Model file for the job. Use its own axes, mm. Face numbers are marked on the shaded views. A direction names the side the tool comes from. Coordinates: 2 decimals unless noted, no trailing zeros. Write each loop counter-clockwise with the first axis right and the second up, starting at its lowest first coordinate (ties: lowest second). Pieces come first, ordered by that corner, then holes.
Q1. Band-saw the part on A-A, the plane z = 1.75. Write the cut outline in (x, y).
Q2. Pull direction X, two halves, no side cores. Call the marked faces 1, 2, 3 and 4: released by +X, released by -X, zero draft, split by the parting line, or undercut.
Q3. Drill centre lines: probe 1 along X at (y, z) = (-16, 3.5); probe 2 along X at (y, z) = (10.5, 2.25); probe 3 along X at (y, z) = (7.5, 5.5). Where is each one in solid material? Low to high.
Q4. Pin check, flat tips, straight feed: P1, Ø1, axis at y = 1, z = 2, coming from the -X side; P2, Ø1.5, axis at x = -30, z = 2.5, coming from the -Y side; P3, Ø4, axis at x = 32, z = 3, coming from the -Y side; P4, Ø21, axis at x = -29.05, y = 0, coming from the +Z side. Stop position of each tip, or through.
Q5. Which spindle directions (+Z, -Z, +X, -X, +Y, -Y) get a long thin tool onto all of the face, cutting with end or side? Do the marked faces 5 and 6. Say none if no direction does.
Q6. Band-saw the part on C-C, the plane y = 0. Write the cut outline in (x, z), plus the area to 3 significant figures.
Q7. Band-saw the part on D-D, the plane x = -17. Write the cut outline in (y, z), plus the area to 3 significant figures.
Q8. Band-saw the part on B-B, the plane x = 35. Write the cut outline in (y, z).
from build123d import *

# Parameters (mm, degrees)
F0_R     = 13.2
F1_DEPTH = 7


with BuildPart() as f1:
    # F0 (on Top) → F1 (new body)
    with BuildSketch(Plane.XY):
        with BuildLine():
            ThreePointArc((5.644667, 22.165649), (4.665852, 19.88717), (3.409515, 17.749143))
            ThreePointArc((3.409515, 17.749143), (0.156216, 19.184844), (-3.20524, 18.024758))
            ThreePointArc((-3.20524, 18.024758), (-4.974394, 19.897283), (-6.195367, 22.165649))
            ThreePointArc((-6.195367, 22.165649), (-7.382922, 19.823517), (-8.993153, 17.749143))
            ThreePointArc((-8.993153, 17.749143), (-22.389875, 12.804904), (-33.179633, 22.158981))
            ThreePointArc((-33.179633, 22.158981), (-49.675616, 1.648765), (-33.179633, -18.861452))
            ThreePointArc((-33.179633, -18.861452), (-15.982306, -11.966628), (0, -21.339599))
            ThreePointArc((0, -21.339599), (18.241916, -11.616609), (36.483832, -21.339599))
            ThreePointArc((36.483832, -21.339599), (50.653593, 0.409691), (36.483832, 22.158981))
            ThreePointArc((36.483832, 22.158981), (23.994879, 12.812003), (9.197427, 17.749143))
            ThreePointArc((9.197427, 17.749143), (7.450629, 19.981192), (5.644667, 22.165649))
        make_face()
        with Locations((-29.049389, 0)):
            Circle(F0_R, mode=Mode.SUBTRACT)
        Circle(F0_R, mode=Mode.SUBTRACT)
        with Locations((29.32474, 0)):
            Circle(F0_R, mode=Mode.SUBTRACT)
    extrude(amount=F1_DEPTH)


solid = f1.part
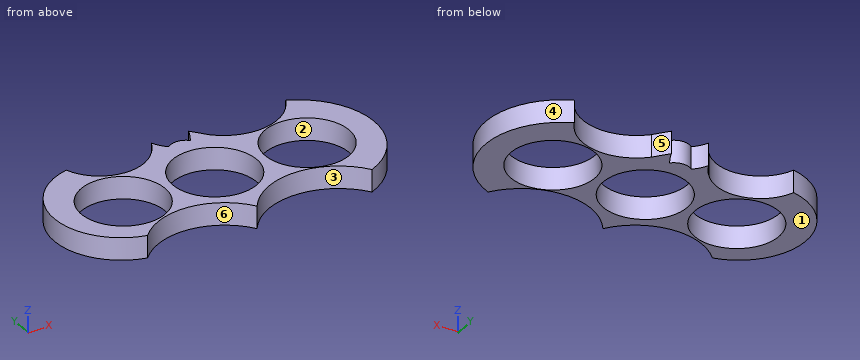
Answer sheet:
1. outline: (-33.18, -18.86) arc R21.04 cw to (0, -21.34) arc R21.97 cw to (36.48, -21.34) arc R23.78 ccw to (36.48, 22.16) arc R16.82 cw to (9.2, 17.75) arc R105.8 ccw to (5.64, 22.17) arc R19.77 cw to (3.41, 17.75) arc R4.87 ccw to (-3.21, 18.02) arc R9.81 cw to (-6.2, 22.17) arc R13.78 cw to (-8.99, 17.75) arc R14.03 cw to (-33.18, 22.16) arc R21 ccw to start; hole circle Ø26.4 at (-29.05, 0); hole circle Ø26.4 at (0, 0); hole circle Ø26.4 at (29.32, 0)
2. face 1: zero draft
2. face 2: undercut
2. face 3: undercut
2. face 4: released by +X
3. probe 1: x = -40.06 to -30.02, -5.08 to 5.07, 31.41 to 44.08
3. probe 2: x = -47.72 to -37.05, -21.05 to -8, 8 to 21.33, 37.32 to 48.41
3. probe 3: x = -48.84 to -39.91, -18.19 to -10.86, 10.86 to 18.46, 40.19 to 49.57
4. P1: stops at x = -49.68
4. P2: stops at y = -16.56
4. P3: stops at y = -18.28
4. P4: passes through
5. face 5: +Z, -Z, +Y
5. face 6: +Z, -Z, -Y
6. outline: (-49.61, 0) - (-42.25, 0) - (-42.25, 7) - (-49.61, 7) - close; (-15.85, 0) - (-13.2, 0) - (-13.2, 7) - (-15.85, 7) - close; (13.2, 0) - (16.12, 0) - (16.12, 7) - (13.2, 7) - close; (42.52, 0) - (50.65, 0) - (50.65, 7) - (42.52, 7) - close
6. area: 147 mm2
7. outline: (-11.92, 0) - (-5.39, 0) - (-5.39, 7) - (-11.92, 7) - close; (5.39, 0) - (12.87, 0) - (12.87, 7) - (5.39, 7) - close
7. area: 98.1 mm2
8. outline: (-19.38, 0) - (-11.92, 0) - (-11.92, 7) - (-19.38, 7) - close; (11.92, 0) - (19.64, 0) - (19.64, 7) - (11.92, 7) - close
